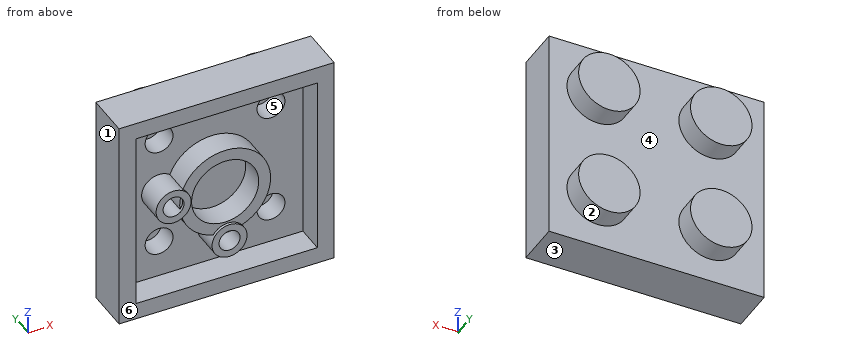
```python
from build123d import *

# Parameters (mm, degrees)
BASEFRAMESKETCH_W           = 15.38
BASEFRAMESKETCH_H           = 3.2
BASEFRAME_DEPTH             = 7.69
STUDSSKETCH_R               = 2.197938665
STUDS_DEPTH                 = 1.6
MAINSTUDSPATTERN_COUNT      = 2
MAINSTUDSPATTERN_PITCH      = 8
MAINSTUDSPATTERN_COUNT_DIR2 = 2
MAINSTUDSPATTERN_PITCH_DIR2 = 8
MAINBASESHELL_T             = -1.2
UNDERCIRCLESKETCH_R         = 3.25
UNDERCIRCLESKETCH_R_2       = 2.4
UNDERCIRCLEEXTRUDE_DEPTH    = 1.8
SMALLUNDERSIDEHOLEX_REACH   = 17.429
HOLEXSKETCH_R               = 1.25
HOLEXSKETCH_R_2             = 0.75
SMALLUNDERSIDEHOLEY_REACH   = 17.429
HOLEYSKETCH_R               = 1.25
HOLEYSKETCH_R_2             = 0.75


with BuildPart() as part:
    # BaseFrameSketch → BaseFrame (new, symmetric)
    with BuildSketch(Plane.XY):
        with Locations((-4.794729064, 1.6)):
            Rectangle(BASEFRAMESKETCH_W, BASEFRAMESKETCH_H)
    extrude(amount=BASEFRAME_DEPTH, both=True)

    # StudsSketch → Studs (add)
    with BuildSketch(Plane(origin=(0, 3.2, 0), x_dir=(1, 0, 0), z_dir=(0, 1, 0))):
        with Locations((-8.584729064, 3.79)):
            Circle(STUDSSKETCH_R)
    studs = extrude(amount=STUDS_DEPTH)

    # MainStudsPattern: Studs 2 × 2
    with Locations(*[(i * MAINSTUDSPATTERN_PITCH, 0, j * MAINSTUDSPATTERN_PITCH_DIR2) for i in range(MAINSTUDSPATTERN_COUNT) for j in range(MAINSTUDSPATTERN_COUNT_DIR2) if (i, j) != (0, 0)]):
        add(studs)

    # MainBaseShell
    mainbaseshell_openings = [part.faces().sort_by_distance(p)[0] for p in [
        (-4.794729064, 0, 0),
    ]]
    offset(amount=MAINBASESHELL_T, openings=mainbaseshell_openings, kind=Kind.INTERSECTION)

    # UnderCircleSketch → UnderCircleExtrude (add)
    with BuildSketch(Plane(origin=(0, 2, 0), x_dir=(-1, 0, 0), z_dir=(0, -1, 0))):
        with Locations(Location((4.794729064, 0, 0), (0, 0, 270))):
            Circle(UNDERCIRCLESKETCH_R)
        with Locations(Location((4.794729064, 0, 0), (0, 0, 270))):
            Circle(UNDERCIRCLESKETCH_R_2, mode=Mode.SUBTRACT)
    extrude(amount=UNDERCIRCLEEXTRUDE_DEPTH)

    # HoleXSketch → SmallUnderSideHoleX (add, up to next)
    with BuildSketch(Plane(origin=(0, 0, 0), x_dir=(-1, 0, 0), z_dir=(0, -1, 0)), mode=Mode.PRIVATE) as smallundersideholex_sk1:
        with Locations(Location((4.584729064, 3.79, 0), (0, 0, 90))):
            Circle(HOLEXSKETCH_R)
        with Locations(Location((4.584729064, 3.79, 0), (0, 0, 90))):
            Circle(HOLEXSKETCH_R_2, mode=Mode.SUBTRACT)
    smallundersideholex_tool1 = extrude(smallundersideholex_sk1.sketch, amount=-SMALLUNDERSIDEHOLEX_REACH, mode=Mode.PRIVATE) - part.part
    add(smallundersideholex_tool1.solids().sort_by_distance((-4.584729, 0, -2.575355))[0])

    # HoleYSketch → SmallUnderSideHoleY (add, up to next)
    with BuildSketch(Plane(origin=(0, 0, 0), x_dir=(-1, 0, 0), z_dir=(0, -1, 0)), mode=Mode.PRIVATE) as smallundersideholey_sk1:
        with Locations(Location((8.584729064, -0.21, 0), (0, 0, 90))):
            Circle(HOLEYSKETCH_R)
        with Locations(Location((8.584729064, -0.21, 0), (0, 0, 90))):
            Circle(HOLEYSKETCH_R_2, mode=Mode.SUBTRACT)
    smallundersideholey_tool1 = extrude(smallundersideholey_sk1.sketch, amount=-SMALLUNDERSIDEHOLEY_REACH, mode=Mode.PRIVATE) - part.part
    add(smallundersideholey_tool1.solids().sort_by_distance((-8.584729, 0, 1.424645))[0])


solid = part.part
```
Design review of the part built by this model. Coordinates are the model's own, in mm. Face numbers are marked on the shaded views. A direction names the side the tool comes from. Coordinates: 2 decimals unless noted, no trailing zeros. Order: outer loops, then holes, each group sorted by start corner. A loop starts at its lowest first (then second) coordinate and runs counter-clockwise, first axis right, second up.
1) Mouldability with a two-part tool opening along X and no side actions: class the marked faces 1, 2 and 3 as +X half, -X half, draft (parallel to the pull), parting line (faces both ways), or undercut.
2) Wall thickness on line 1 along Z through (x, y) = (0, 0.4); line 2 along Z through (x, y) = (-8.75, 1.1); line 3 along X through (y, z) = (1.8, 6): over which ranges is each line inside the solid? List them lowest first.
3) For the marked faces 4, 5 and 6, list the 3-axis set-ups (+Z, -Z, +X, -X, +Y, -Y) from which the entire face can be reached by the end or side of a thin tool; tool diameter is ignored.
4) Take a section at B-B, the plane y = 2.6. Give the boundary of the cut face in (x, z), and give its area (3 significant figures).
5) Clearance check with flat-ended pins moving along their axes: pin 1 (0.9 mm diameter, centred on x = -8.58, z = 0.21, fed in from +Y); pin 2 (3 mm diameter, centred on x = -4.79, z = 0, fed in from -Y); pin 3 (1 mm diameter, centred on x = -8.5, y = 4, fed in from +Z). State where each tip first meets the part, or that it passes through.
6) Take a section at A-A, the plane y = 1.8. Give the boundary of the cut face in (x, z), and give its area (3 significant figures).
7) Take a section at D-D, the plane x = -1.25. Give the boundary of the cut face in (y, z), and give its area (3 significant figures).
Returned:
1. face 1: -X half
1. face 2: undercut
1. face 3: draft
2. line 1: z = -7.69 to -6.49, 6.49 to 7.69
2. line 2: z = -7.69 to -6.49, -1.03 to -0.52, 0.94 to 1.45, 6.49 to 7.69
2. line 3: x = -12.48 to -11.28, 1.7 to 2.9
3. face 4: +Y
3. face 5: -Y
3. face 6: +Z, -Z, +X, -X, -Y
4. outline: (-12.48, -7.69) - (2.9, -7.69) - (2.9, 7.69) - (-12.48, 7.69) - close; hole circle Ø2 at (-8.58, -3.79); hole circle Ø2 at (-8.58, 4.21); hole circle Ø2 at (-0.58, -3.79); hole circle Ø2 at (-0.58, 4.21)
4. area: 224 mm2
5. pin 1: stops at y = 3.2
5. pin 2: stops at y = 2
5. pin 3: stops at z = 6.41
6. outline: (-12.48, -7.69) - (2.9, -7.69) - (2.9, 7.69) - (-12.48, 7.69) - close; (-7.93, -0.85) arc R3.25 ccw to (-5.65, -3.14) arc R1.25 ccw (long way) to (-3.6, -3.02) arc R3.25 ccw (long way) to (-7.82, 1.2) arc R1.25 ccw (long way) to start; hole (-11.28, -6.49) - (1.7, -6.49) - (1.7, 6.49) - (-11.28, 6.49) - close; hole (-8.03, -0.3) arc R3.25 cw to (-7.98, 0.65) arc R0.75 ccw (long way) to start; hole circle Ø4.8 at (-4.79, 0); hole (-5.09, -3.24) arc R0.75 ccw (long way) to (-4.14, -3.18) arc R3.25 cw to start
6. area: 87.7 mm2
7. outline: (0, -7.69) - (3.2, -7.69) - (3.2, -5.88) - (4.8, -5.88) - (4.8, -1.7) - (3.2, -1.7) - (3.2, 2.12) - (4.8, 2.12) - (4.8, 6.3) - (3.2, 6.3) - (3.2, 7.69) - (0, 7.69) - (0, 6.49) - (2, 6.49) - (2, 4.95) - (3.6, 4.95) - (3.6, 3.47) - (2, 3.47) - (2, -3.05) - (3.6, -3.05) - (3.6, -4.53) - (2, -4.53) - (2, -6.49) - (0, -6.49) - close
7. area: 31.9 mm2
